Here's how the part is built. I have some questions about the finished solid (model axes, mm). A direction names the side the tool comes from. Coordinates: 2 decimals unless noted, no trailing zeros. Loops run counter-clockwise (first coordinate to the right, second up) from the corner with the lowest first, then second, coordinate; pieces in that order, holes last.
from build123d import *

# Parameters (mm, degrees)
SKETCH1_W           = 43
SKETCH1_H           = 13.5
SKETCH4_R           = 6
BOSS_EXTRUDE2_DEPTH = 20
SKETCH5_R           = 6
BOSS_EXTRUDE3_DEPTH = 18
FILLET1_R           = 6
SKETCH6_R           = 6
BOSS_EXTRUDE4_DEPTH = 18
FILLET2_R           = 6
FILLET3_R           = 2
SKETCH8_W           = 43
SKETCH8_H           = 23
CUT_EXTRUDE2_DEPTH  = 7
SKETCH9_W           = 43
SKETCH9_H           = 23
SKETCH9_R           = 6
CUT_EXTRUDE3_DEPTH  = 5


with BuildPart() as part:
    # Sketch1 → Revolve1 (revolve)
    with BuildSketch(Plane(origin=(0, 0, 0), x_dir=(1, 0, 0), z_dir=(0, 1, 0))):
        with Locations((-25.810870043, -6.75)):
            Rectangle(SKETCH1_W, SKETCH1_H)
    revolve(axis=Axis((-47.310870043, 0, 0), (1, 0, 0)))

    # Sketch4 → Boss-Extrude2 (add)
    with BuildSketch(Plane.XY):
        with Locations((-37.310870043, 0)):
            Circle(SKETCH4_R)
    extrude(amount=BOSS_EXTRUDE2_DEPTH)

    # Sketch5 → Boss-Extrude3 (add)
    with BuildSketch(Plane.ZY.offset(47.310870043)):
        Circle(SKETCH5_R)
    extrude(amount=BOSS_EXTRUDE3_DEPTH)

    # Fillet1
    fillet1_edges = [part.edges().sort_by_distance(p)[0] for p in [
        (-65.310870043, 0, -6),
    ]]
    fillet(fillet1_edges, radius=FILLET1_R)

    # Sketch6 → Boss-Extrude4 (add)
    with BuildSketch(Plane(origin=(-4.310870043, 0, 0), x_dir=(0, 0, -1), z_dir=(1, 0, 0))):
        Circle(SKETCH6_R)
    extrude(amount=BOSS_EXTRUDE4_DEPTH)

    # Fillet2
    fillet2_edges = [part.edges().sort_by_distance(p)[0] for p in [
        (13.689129957, 0, 6),
    ]]
    fillet(fillet2_edges, radius=FILLET2_R)

    # Fillet3
    fillet3_edges = [part.edges().sort_by_distance(p)[0] for p in [
        (-4.310870043, 0, -13.5),
        (-47.310870043, 0, -13.5),
    ]]
    fillet(fillet3_edges, radius=FILLET3_R)

    # Sketch8 → Cut-Extrude2 (cut)
    with BuildSketch(Plane.XY.offset(-12)):
        with Locations((-25.810870043, 0)):
            Rectangle(SKETCH8_W, SKETCH8_H)
    extrude(amount=-CUT_EXTRUDE2_DEPTH, mode=Mode.SUBTRACT)

    # Sketch9 → Cut-Extrude3 (cut)
    with BuildSketch(Plane.XY.offset(12)):
        with Locations((-25.810870043, 0)):
            Rectangle(SKETCH9_W, SKETCH9_H)
        with Locations((-37.310870043, 0)):
            Circle(SKETCH9_R, mode=Mode.SUBTRACT)
    extrude(amount=CUT_EXTRUDE3_DEPTH, mode=Mode.SUBTRACT)


solid = part.part
Q1. Will these pins go through, and if not, where does the flat tip stop? P1, Ø5, axis at x = -54, y = -2, coming from the -Z side; P2, Ø3.5, axis at x = -27, y = 2.5, coming from the +Z side; P3, Ø2, axis at y = -9.5, z = 0, coming from the -X side.
Q2. Suppose I cut it at A-A on y = 0. Write out the boundary of the cut face in (x, z), and give its area (3 significant figures).
Q3. Suppose I cut it at C-C on x = -57. Write out the boundary of the cut face in (y, z), and give its area (3 significant figures).
Q4. Suppose I cut it at B-B on z = 0. Write out the boundary of the cut face in (x, y).
Q5. For faces 1 (the cylindrical face through (-53, 0, -6)), 2 (the cylindrical face through (2, 0, 6)), 3 (the flat face through (-37, 0, 20)), which set-ups out of +Z, -Z, +X, -X, +Y, -Y let a thin tool reach every point of the face, with its end or its side?
Q6. Suppose I cut it at D-D on x = -10. Write out the boundary of the cut face in (y, z).
Q7. Please list where these lines run through material, in increasing order: probe 1 along Z at (x, y) = (-31, 4); probe 2 along X at (y, z) = (7.75, -1.5); probe 3 along Y at (x, z) = (-9.5, -1.5).
Check values:
1. P1: stops at z = -6
1. P2: stops at z = 12
1. P3: stops at x = -47.31
2. outline: (-59.31, -6) - (-47.31, -6) - (-47.31, -11.5) arc R2 ccw to (-47.25, -12) - (-4.37, -12) arc R2 ccw to (-4.31, -11.5) - (-4.31, -6) - (7.69, -6) arc R6 ccw to (7.69, 6) - (-4.31, 6) - (-4.31, 11.5) arc R2 ccw to (-4.37, 12) - (-31.31, 12) - (-31.31, 20) - (-43.31, 20) - (-43.31, 12) - (-47.25, 12) arc R2 ccw to (-47.31, 11.5) - (-47.31, 6) - (-59.31, 6) arc R6 ccw to start
2. area: 1,530 mm2
3. outline: circle Ø12 at (0, 0)
3. area: 113 mm2
4. outline: (-59.31, -6) - (-47.31, -6) - (-47.31, -11.5) arc R2 ccw to (-45.31, -13.5) - (-6.31, -13.5) arc R2 ccw to (-4.31, -11.5) - (-4.31, -6) - (7.69, -6) arc R6 ccw to (7.69, 6) - (-4.31, 6) - (-4.31, 11.5) arc R2 ccw to (-6.31, 13.5) - (-45.31, 13.5) arc R2 ccw to (-47.31, 11.5) - (-47.31, 6) - (-59.31, 6) arc R6 ccw to start
5. face 1: -X
5. face 2: +X
5. face 3: +Z, +X, -X, +Y, -Y
6. outline: (-6.18, -12) - (6.18, -12) arc R13.5 ccw to (6.18, 12) - (-6.18, 12) arc R13.5 ccw to start
7. probe 1: z = -12 to 12
7. probe 2: x = -47.31 to -4.31
7. probe 3: y = -13.42 to 13.42
